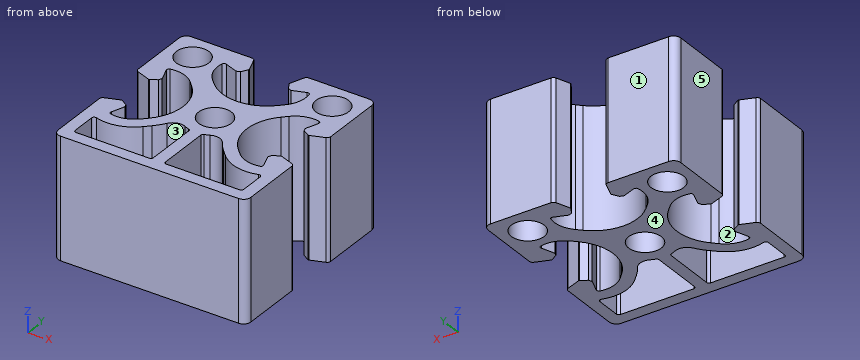
```python
from build123d import *

# Parameters (mm, degrees)
SK_MAIN_EXTRUSION_R  = 3.4
MAIN_EXTRUSION_DEPTH = 25


with BuildPart() as part:
    # Sk Main Extrusion → Main Extrusion (new body)
    with BuildSketch(Plane.XY):
        with BuildLine():
            Line((-16.671180212, -4.190076845), (-19.506515107, -5.222054351))
            ThreePointArc((-19.506515107, -5.222054351), (-19.864364033, -5.496641489), (-20, -5.926823816))
            Line((-20, -5.926823816), (-20, -18.5))
            ThreePointArc((-20, -18.5), (-19.560660172, -19.560660172), (-18.5, -20))
            Line((-18.5, -20), (18.5, -20))
            ThreePointArc((18.5, -20), (19.560660172, -19.560660172), (20, -18.5))
            Line((20, -18.5), (20, -5.926823816))
            ThreePointArc((20, -5.926823816), (19.864364033, -5.496641489), (19.506515107, -5.222054351))
            Line((19.506515107, -5.222054351), (16.671180212, -4.190076845))
            ThreePointArc((16.671180212, -4.190076845), (16.563886241, -4.175951325), (16.460675177, -4.208493649))
            Line((16.460675177, -4.208493649), (15.111296024, -4.987558066))
            Line((15.111296024, -4.987558066), (14.845251581, -5.718509166))
            Line((14.845251581, -5.718509166), (15.81984631, -8.396186179))
            ThreePointArc((15.81984631, -8.396186179), (15.786489799, -8.811074612), (15.450654467, -9.056960151))
            ThreePointArc((15.450654467, -9.056960151), (12.665882372, -8.933433013), (10.272684887, -7.504160339))
            Line((10.272684887, -7.504160339), (9.309262274, -6.540737726))
            ThreePointArc((9.309262274, -6.540737726), (6.6, 0), (9.309262274, 6.540737726))
            Line((9.309262274, 6.540737726), (10.272684887, 7.504160339))
            ThreePointArc((10.272684887, 7.504160339), (12.665882372, 8.933433013), (15.450654467, 9.056960151))
            ThreePointArc((15.450654467, 9.056960151), (15.786489799, 8.811074612), (15.81984631, 8.396186179))
            Line((15.81984631, 8.396186179), (14.845251581, 5.718509166))
            Line((14.845251581, 5.718509166), (15.111296024, 4.987558066))
            Line((15.111296024, 4.987558066), (16.460675177, 4.208493649))
            ThreePointArc((16.460675177, 4.208493649), (16.563886241, 4.175951325), (16.671180212, 4.190076845))
            Line((16.671180212, 4.190076845), (19.506515107, 5.222054351))
            ThreePointArc((19.506515107, 5.222054351), (19.864364033, 5.496641489), (20, 5.926823816))
            Line((20, 5.926823816), (20, 18.5))
            ThreePointArc((20, 18.5), (19.560660172, 19.560660172), (18.5, 20))
            Line((18.5, 20), (5.926823816, 20))
            ThreePointArc((5.926823816, 20), (5.496641489, 19.864364033), (5.222054351, 19.506515107))
            Line((5.222054351, 19.506515107), (4.190076845, 16.671180212))
            ThreePointArc((4.190076845, 16.671180212), (4.175951325, 16.563886241), (4.208493649, 16.460675177))
            Line((4.208493649, 16.460675177), (4.987558066, 15.111296024))
            Line((4.987558066, 15.111296024), (5.718509166, 14.845251581))
            Line((5.718509166, 14.845251581), (8.396186179, 15.81984631))
            ThreePointArc((8.396186179, 15.81984631), (8.811074612, 15.786489799), (9.056960151, 15.450654467))
            ThreePointArc((9.056960151, 15.450654467), (8.933433013, 12.665882372), (7.504160339, 10.272684887))
            Line((7.504160339, 10.272684887), (6.540737726, 9.309262274))
            ThreePointArc((6.540737726, 9.309262274), (0, 6.6), (-6.540737726, 9.309262274))
            Line((-6.540737726, 9.309262274), (-7.504160339, 10.272684887))
            ThreePointArc((-7.504160339, 10.272684887), (-8.933433013, 12.665882372), (-9.056960151, 15.450654467))
            ThreePointArc((-9.056960151, 15.450654467), (-8.811074612, 15.786489799), (-8.396186179, 15.81984631))
            Line((-8.396186179, 15.81984631), (-5.718509166, 14.845251581))
            Line((-5.718509166, 14.845251581), (-4.987558066, 15.111296024))
            Line((-4.987558066, 15.111296024), (-4.208493649, 16.460675177))
            ThreePointArc((-4.208493649, 16.460675177), (-4.175951325, 16.563886241), (-4.190076845, 16.671180212))
            Line((-4.190076845, 16.671180212), (-5.222054351, 19.506515107))
            ThreePointArc((-5.222054351, 19.506515107), (-5.496641489, 19.864364033), (-5.926823816, 20))
            Line((-5.926823816, 20), (-18.5, 20))
            ThreePointArc((-18.5, 20), (-19.560660172, 19.560660172), (-20, 18.5))
            Line((-20, 18.5), (-20, 5.926823816))
            ThreePointArc((-20, 5.926823816), (-19.864364033, 5.496641489), (-19.506515107, 5.222054351))
            Line((-19.506515107, 5.222054351), (-16.671180212, 4.190076845))
            ThreePointArc((-16.671180212, 4.190076845), (-16.563886241, 4.175951325), (-16.460675177, 4.208493649))
            Line((-16.460675177, 4.208493649), (-15.111296024, 4.987558066))
            Line((-15.111296024, 4.987558066), (-14.845251581, 5.718509166))
            Line((-14.845251581, 5.718509166), (-15.81984631, 8.396186179))
            ThreePointArc((-15.81984631, 8.396186179), (-15.786489799, 8.811074612), (-15.450654467, 9.056960151))
            ThreePointArc((-15.450654467, 9.056960151), (-12.665882372, 8.933433013), (-10.272684887, 7.504160339))
            Line((-10.272684887, 7.504160339), (-9.309262274, 6.540737726))
            ThreePointArc((-9.309262274, 6.540737726), (-6.6, 0), (-9.309262274, -6.540737726))
            Line((-9.309262274, -6.540737726), (-10.272684887, -7.504160339))
            ThreePointArc((-10.272684887, -7.504160339), (-12.665882372, -8.933433013), (-15.450654467, -9.056960151))
            ThreePointArc((-15.450654467, -9.056960151), (-15.786489799, -8.811074612), (-15.81984631, -8.396186179))
            Line((-15.81984631, -8.396186179), (-14.845251581, -5.718509166))
            Line((-14.845251581, -5.718509166), (-15.111296024, -4.987558066))
            Line((-15.111296024, -4.987558066), (-16.460675177, -4.208493649))
            ThreePointArc((-16.460675177, -4.208493649), (-16.563886241, -4.175951325), (-16.671180212, -4.190076845))
        make_face()
        with Locations((14.5, 14.5)):
            Circle(SK_MAIN_EXTRUSION_R, mode=Mode.SUBTRACT)
        Circle(SK_MAIN_EXTRUSION_R, mode=Mode.SUBTRACT)
        with Locations((-14.5, 14.5)):
            Circle(SK_MAIN_EXTRUSION_R, mode=Mode.SUBTRACT)
        with BuildLine():
            Line((-7.441495321, -8.308504679), (-8.577273231, -9.444282589))
            ThreePointArc((-8.577273231, -9.444282589), (-12.430514315, -11.611987193), (-16.849169473, -11.464011904))
            ThreePointArc((-16.849169473, -11.464011904), (-17.295452819, -11.537349181), (-17.5, -11.940719521))
            Line((-17.5, -11.940719521), (-17.5, -17))
            ThreePointArc((-17.5, -17), (-17.353553391, -17.353553391), (-17, -17.5))
            Line((-17, -17.5), (-1.75, -17.5))
            ThreePointArc((-1.75, -17.5), (-1.396446609, -17.353553391), (-1.25, -17))
            Line((-1.25, -17), (-1.25, -6.156094541))
            ThreePointArc((-1.25, -6.156094541), (-1.351026708, -5.854730455), (-1.61328125, -5.675149655))
            ThreePointArc((-1.61328125, -5.675149655), (-2.10305366, -5.51245547), (-2.576734694, -5.307583096))
            ThreePointArc((-2.576734694, -5.307583096), (-4.359333373, -5.153883821), (-5.788120301, -6.230846881))
            ThreePointArc((-5.788120301, -6.230846881), (-6.555931161, -7.316529108), (-7.441495321, -8.308504679))
        make_face(mode=Mode.SUBTRACT)
        with BuildLine():
            Line((1.25, -6.156094541), (1.25, -17))
            ThreePointArc((1.25, -17), (1.396446609, -17.353553391), (1.75, -17.5))
            Line((1.75, -17.5), (17, -17.5))
            ThreePointArc((17, -17.5), (17.353553391, -17.353553391), (17.5, -17))
            Line((17.5, -17), (17.5, -11.940719521))
            ThreePointArc((17.5, -11.940719521), (17.295452819, -11.537349181), (16.849169473, -11.464011904))
            ThreePointArc((16.849169473, -11.464011904), (12.430514315, -11.611987193), (8.577273231, -9.444282589))
            Line((8.577273231, -9.444282589), (7.441495321, -8.308504679))
            ThreePointArc((7.441495321, -8.308504679), (6.555931161, -7.316529108), (5.788120301, -6.230846881))
            ThreePointArc((5.788120301, -6.230846881), (4.359333373, -5.153883821), (2.576734694, -5.307583096))
            ThreePointArc((2.576734694, -5.307583096), (2.10305366, -5.51245547), (1.61328125, -5.675149655))
            ThreePointArc((1.61328125, -5.675149655), (1.351026708, -5.854730455), (1.25, -6.156094541))
        make_face(mode=Mode.SUBTRACT)
    extrude(amount=-MAIN_EXTRUSION_DEPTH)


solid = part.part
```
Can you work these out from the model? Positions are in its coordinate system, mm. Face numbers are marked on the shaded views. A direction names the side the tool comes from. Give positions to 0.01 mm unless a question says otherwise; leave off trailing zeros. Order: outer loops, then holes, each group sorted by start corner. A loop starts at its lowest first (then second) coordinate and runs counter-clockwise, first axis right, second up. Notation, with made-up numbers: M 64.25,53 L 117.25,53 A16 cw 117.25,61 Z; hole C 18,81 d1. An arc over 180 degrees is marked long. Write item = value, one per line. Start each with the question number.
Q1. Will this pin go through, and if not, where does the flat tip stop? pin 1 Ø6 at (y, z) = (-2.5, -8.5) entering from +X.
Q2. Suppose I cut it at D-D (x = -12). Write out the boundary of the cut face in (y, z).
Q3. Suppose I cut it at A-A (y = 0). Write out the boundary of the cut face in (x, z).
Q4. Suppose I cut it at B-B (x = 0). Write out the boundary of the cut face in (y, z).
Q5. Suppose I cut it at C-C (y = -14). Write out the boundary of the cut face in (x, z).
Q6. I need wall thicknesses on probe 1 along Y at (x, z) = (-14.5, -8); probe 2 along Y at (x, z) = (0, -12.5); probe 3 along X at (y, z) = (-15, -4.75). Which ranges of each line are inside material? Lowest first, please. Write a range as [from, to].
Q7. We'd pull the mould along X, two halves only. Please class the marked faces 3, 4 and 5: pulls with the +X half, pulls with the -X half, needs draft (parallel to the pull), parting line crosses it, or undercut.
Q8. For the marked faces 1 and 2, which set-ups out of +Z, -Z, +X, -X, +Y, -Y let a thin tool reach every point of the face, with its end or its side?
Check result:
q1.pin_1 = 19.87
q2.outline = M -20,-25 L -17.5,-25 L -17.5,0 L -20,0 Z; M -11.49,-25 L -8.69,-25 L -8.69,0 L -11.49,0 Z; M 8.69,-25 L 12.2,-25 L 12.2,0 L 8.69,0 Z; M 16.8,-25 L 20,-25 L 20,0 L 16.8,0 Z
q3.outline = M -6.6,-25 L -3.4,-25 L -3.4,0 L -6.6,0 Z; M 3.4,-25 L 6.6,-25 L 6.6,0 L 3.4,0 Z
q4.outline = M -20,-25 L -3.4,-25 L -3.4,0 L -20,0 Z; M 3.4,-25 L 6.6,-25 L 6.6,0 L 3.4,0 Z
q5.outline = M -20,-25 L -17.5,-25 L -17.5,0 L -20,0 Z; M -1.25,-25 L 1.25,-25 L 1.25,0 L -1.25,0 Z; M 17.5,-25 L 20,-25 L 20,0 L 17.5,0 Z
q6.probe_1 = [-20, -17.5], [-11.85, -9.17], [9.17, 11.1], [17.9, 20]
q6.probe_2 = [-20, -3.4], [3.4, 6.6]
q6.probe_3 = [-20, -17.5], [-1.25, 1.25], [17.5, 20]
q7.face_3 = undercut
q7.face_4 = needs draft
q7.face_5 = pulls with the -X half
q8.face_1 = +Z, -Z, +X, -X, +Y
q8.face_2 = +Z, -Z
